The model under review builds one solid part; all positions refer to its coordinate system, in mm. Round coordinates to 2 decimals unless told otherwise and drop trailing zeros. Order: outer loops, then holes, each group sorted by start corner. A loop starts at its lowest first (then second) coordinate and runs counter-clockwise, first axis right, second up. Notation, with made-up numbers: M 44.25,58 L 56.25,58 A20 ccw 56.25,86 Z; hole C 14,45.25 d11. An arc over 180 degrees is marked long. Answer as a JSON object with one key per item and string values. Group by question number.
1) Consider section C-C, the plane y = 157. Write out the cut boundary in (x, z), then the cut area to 3 significant figures.
2) Consider section A-A, the plane x = 2.9. Write out the cut boundary in (y, z).
3) Insertion check: pin 1 Ø3 at (y, z) = (69.85, -49.11) entering from +X. The pin has a flat end and moves straight along its axis. Give the tip position at first contact, or say it passes through.
4) Consider section B-B, the plane z = 28.5. Write out the cut boundary in (x, y).
5) To check wall thickness, follow line 1 (Z direction, x = 0.65, y = 206.5); line 2 (Z direction, x = 1.8, y = 69.85); line 3 (Z direction, x = 0.5, y = 95). State the ranges of each line that lie inside material, in increasing order.
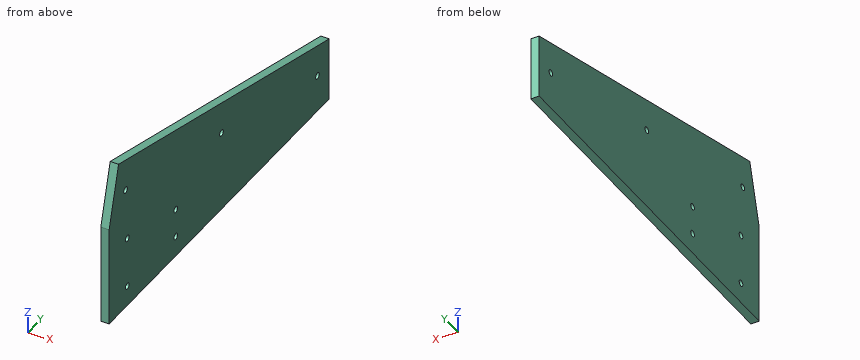
```python
from build123d import *

# Parameters (mm, degrees)
BOSS_EXTRUDE1_DEPTH   = 5.08
F_6_CLEARANCE_HOLE1_D = 3.7973


with BuildPart() as part:
    # Sketch1 → Boss-Extrude1 (new body)
    with BuildSketch(Plane(origin=(0, 0, 0), x_dir=(0, 0, -1), z_dir=(1, 0, 0))):
        Polygon((0, 0), (-36.801773982, 9.861005618), (22.364259729, 230.671649508), (61.808282202, 230.671649508), (61.808282202, 0), align=None)
    extrude(amount=BOSS_EXTRUDE1_DEPTH)

    # #6 Clearance Hole1 (through all)
    with Locations(Plane(origin=(5.08, 0, 0), x_dir=(0, 0, -1), z_dir=(1, 0, 0))):
        with Locations((49.108282202, 69.85), (38.799269093, 218.404391514), (11.842691987, 117.801076159), (-15.113885118, 17.197760803), (49.108282202, 19.05), (17.804432116, 19.05), (31.416251091, 69.85)):
            Hole(F_6_CLEARANCE_HOLE1_D / 2)


solid = part.part
```
Results list:
{
 "1": {"outline": "M 0,-61.81 L 5.08,-61.81 L 5.08,-2.62 L 0,-2.62 Z", "area": "301 mm^2"},
 "2": {"outline": "M 0,-61.81 L 230.67,-61.81 L 230.67,-22.36 L 9.86,36.8 L 0,0 Z; hole C 17.2,15.11 d3.8; hole C 19.05,-49.11 d3.8; hole C 19.05,-17.8 d3.8; hole C 69.85,-49.11 d3.8; hole C 69.85,-31.42 d3.8; hole C 117.8,-11.84 d3.8; hole C 218.4,-38.8 d3.8"},
 "3": {"pin 1": "through"},
 "4": {"outline": "M 0,7.64 L 5.08,7.64 L 5.08,40.84 L 0,40.84 Z"},
 "5": {"line 1": "-61.81 to -15.89", "line 2": "-61.81 to -51.01, -47.21 to -33.31, -29.52 to 20.73", "line 3": "-61.81 to 13.99"}
}
